from build123d import *

# Parameters (mm, degrees)
F1_DEPTH = 161.925


with BuildPart() as f1:
    # F0 (on Front) → F1 (new body, symmetric)
    with BuildSketch(Plane.XZ):
        with BuildLine():
            ThreePointArc((-13.5001, 1.99898), (-12.914612, 0.585488), (-11.50112, 0))
            Line((-11.50112, 0), (11.50112, 0))
            ThreePointArc((11.50112, 0), (12.914612, 0.585488), (13.5001, 1.99898))
            Line((13.5001, 1.99898), (13.5001, 5.4991))
            ThreePointArc((13.5001, 5.4991), (13.793216, 6.206744), (14.50086, 6.49986))
            Line((14.50086, 6.49986), (18.328109, 6.49986))
            Line((18.328109, 6.49986), (18.328109, 7.50062))
            Line((18.328109, 7.50062), (14.5161, 7.50062))
            ThreePointArc((14.5161, 7.50062), (13.102608, 6.915132), (12.51712, 5.50164))
            Line((12.51712, 5.50164), (12.51712, 2.00152))
            ThreePointArc((12.51712, 2.00152), (12.224004, 1.293876), (11.51636, 1.00076))
            Line((11.51636, 1.00076), (-11.48334, 1.00076))
            ThreePointArc((-11.48334, 1.00076), (-12.190984, 1.293876), (-12.4841, 2.00152))
            Line((-12.4841, 2.00152), (-12.4841, 5.50164))
            ThreePointArc((-12.4841, 5.50164), (-13.069588, 6.915132), (-14.48308, 7.50062))
            Line((-14.48308, 7.50062), (-16.673091, 7.50062))
            Line((-16.673091, 7.50062), (-16.673091, 6.49986))
            Line((-16.673091, 6.49986), (-14.50086, 6.49986))
            ThreePointArc((-14.50086, 6.49986), (-13.793216, 6.206744), (-13.5001, 5.4991))
            Line((-13.5001, 5.4991), (-13.5001, 1.99898))
        make_face()
    extrude(amount=F1_DEPTH, both=True)


solid = f1.part
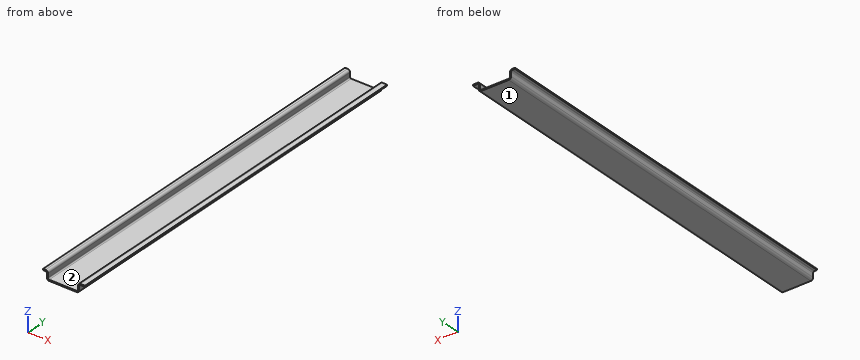
Geometry check sheet. Reference: the model listing, model coordinates, mm. Face numbers are marked on the shaded views. Give positions to 0.01 mm unless a question says otherwise; leave off trailing zeros. Order: outer loops, then holes, each group sorted by start corner. A loop starts at its lowest first (then second) coordinate and runs counter-clockwise, first axis right, second up. Notation, with made-up numbers: (32, 35.5) - (63, 35.5) arc R20 ccw to (63, 55.5) - close; hole circle Ø11 at (79.25, 7.25). An arc over 180 degrees is marked (long way). Use one line per item in the form item = value.
1) Sectioned sample at B-B (z = 3.25). Record the boundary of the cut face in (x, y) (3 decimals).
Working result:
outline = (-13.5, -161.925) - (-12.484, -161.925) - (-12.484, 161.925) - (-13.5, 161.925) - close; (12.517, -161.925) - (13.5, -161.925) - (13.5, 161.925) - (12.517, 161.925) - close
2) Draft check along X on the marked faces 1 and 2. Enter one of: released by +X, released by -X, zero draft, split by the parting line, or undercut.
Working result:
face_1 = zero draft
face_2 = undercut
3) Material ranges on probe 1 along X at (y, z) = (36.5, 4.5); probe 2 along X at (y, z) = (-37, 7.25); probe 3 along Z at (x, y) = (-7, 134), recorded low to high. Write a range as from..to.
Working result:
probe_1 = -13.5..-12.48, 12.52..13.5
probe_2 = -16.67..-13.51, 13.55..18.33
probe_3 = 0..1
4) Sectioned sample at A-A (y = 63). Record the boundary of the cut face in (x, z).
Working result:
outline = (-16.67, 6.5) - (-14.5, 6.5) arc R1 cw to (-13.5, 5.5) - (-13.5, 2) arc R2 ccw to (-11.5, 0) - (11.5, 0) arc R2 ccw to (13.5, 2) - (13.5, 5.5) arc R1 cw to (14.5, 6.5) - (18.33, 6.5) - (18.33, 7.5) - (14.52, 7.5) arc R2 ccw to (12.52, 5.5) - (12.52, 2) arc R1 cw to (11.52, 1) - (-11.48, 1) arc R1 cw to (-12.48, 2) - (-12.48, 5.5) arc R2 ccw to (-14.48, 7.5) - (-16.67, 7.5) - close
5) Depth check by flat-ended pin: pin 1 Ø12 at (x, y) = (8, 97.5) entering from +Z; pin 2 Ø3 at (y, z) = (61, 3.5) entering from +X; pin 3 Ø11.5 at (x, y) = (-3, -47) entering from +Z. Enter the tip coordinate at first touch or a pass-through.
Working result:
pin_1 = 7.43
pin_2 = 13.5
pin_3 = 1
6) Sectioned sample at C-C (x = -4). Record the boundary of the cut face in (y, z) (3 decimals), and give its area (3 significant figures).
Working result:
outline = (-161.925, 0) - (161.925, 0) - (161.925, 1.001) - (-161.925, 1.001) - close
area = 324 mm^2
